Verification items for the finished model (mm, model axes). A direction names the side the tool comes from. Round coordinates to 2 decimals unless told otherwise and drop trailing zeros. Write each loop counter-clockwise with the first axis right and the second up, starting at its lowest first coordinate (ties: lowest second). Pieces come first, ordered by that corner, then holes. Notation, with made-up numbers: M 27,13.25 L 33,13.25 A24 ccw 33,42.25 Z; hole C 37.25,54.25 d1. An arc over 180 degrees is marked long. Answer in a Markdown table with one row per item. Add a question column.
1. Sectioned sample at B-B on z = 0. Record the cut outline in (x, y), plus the area to 3 significant figures.
2. Sectioned sample at A-A on y = 13.5. Record the cut outline in (x, z).
3. Sectioned sample at D-D on z = -7.5. Record the cut outline in (x, y), plus the area to 3 significant figures.
4. Sectioned sample at C-C on x = 0. Record the cut outline in (y, z), plus the area to 3 significant figures.
5. Go/stop test with flat-tipped pins: pin 1 Ø8 at (y, z) = (16.5, -6) entering from -X; pin 2 Ø1.6 at (y, z) = (15, 19.5) entering from +X; pin 3 Ø5 at (x, y) = (-17, 12) entering from +Z; pin 4 Ø12 at (x, z) = (6.5, -10) entering from -Y. Record where each tip stops, or that it passes through.
6. Material ranges on probe 1 along X at (y, z) = (31.05, 0); probe 2 along X at (y, z) = (8.5, 0); probe 3 along X at (y, z) = (25, 2.5), recorded low to high.
7. Set-up check for faces 1 (the flat face through (0, 0, 0)), 2 (the flat face through (-6, 16, 13.16)), 3 (the flat face through (-4.28, 30, 20)): record each of +Z, -Z, +X, -X, +Y, -Y from which the full face is reachable in a straight line by a thin tool's end or side.
8. Draft check along Z on faces 4 (the flat face through (0, 16, 21.46)), 5 (the flat face through (0, 27.573, 20)), 6 (the cylindrical face through (0.642, 16.993, -14.586)). Enter one of: pulls with the +Z half, pulls with the -Z half, needs draft (parallel to the pull), parting line crosses it, or undercut.
```python
from build123d import *

# Parameters (mm, degrees)
SKETCH1_R           = 17
BOSS_EXTRUDE1_DEPTH = 32
SHELL1_T            = -2.4
SKETCH2_R           = 3.45
BOSS_EXTRUDE3_DEPTH = 3
SKETCH4_R           = 2.25
CUT_EXTRUDE1_DEPTH  = 3
SKETCH5_W           = 12.1
SKETCH5_H           = 8.3
BOSS_EXTRUDE4_DEPTH = 26
SKETCH6_W           = 10.4
SKETCH6_H           = 8.6
CUT_EXTRUDE2_DEPTH  = 25
SKETCH7_W           = 8.6
SKETCH7_H           = 5.8
CUT_EXTRUDE3_DEPTH  = 5


with BuildPart() as part:
    # Sketch1 → Boss-Extrude1 (new body)
    with BuildSketch(Plane(origin=(0, 0, 0), x_dir=(1, 0, 0), z_dir=(0, 1, 0))):
        with Locations(Location((0, 0, 0), (0, 0, 270))):
            Circle(SKETCH1_R)
    extrude(amount=BOSS_EXTRUDE1_DEPTH)

    # Shell1
    shell1_openings = [part.faces().sort_by_distance(p)[0] for p in [
        (0, 32, 0),
    ]]
    offset(amount=SHELL1_T, openings=shell1_openings, kind=Kind.INTERSECTION)

    # Sketch2 → Boss-Extrude3 (add)
    with BuildSketch(Plane(origin=(0, 32, 0), x_dir=(1, 0, 0), z_dir=(0, 1, 0))):
        with Locations((18.659372003, 0)):
            Circle(SKETCH2_R)
        with Locations((-18.659372003, 0)):
            Circle(SKETCH2_R)
    extrude(amount=-BOSS_EXTRUDE3_DEPTH)

    # Sketch4 → Cut-Extrude1 (cut)
    with BuildSketch(Plane(origin=(0, 32, 0), x_dir=(1, 0, 0), z_dir=(0, 1, 0))):
        with Locations(Location((18.946509427, 0, 0), (0, 0, 270))):
            Circle(SKETCH4_R)
        with Locations(Location((-18.946509427, 0, 0), (0, 0, 331.648790534))):
            Circle(SKETCH4_R)
    extrude(amount=-CUT_EXTRUDE1_DEPTH, mode=Mode.SUBTRACT)

    # Sketch5 → Boss-Extrude4 (add)
    with BuildSketch(Plane(origin=(0, 32, 0), x_dir=(1, 0, 0), z_dir=(0, 1, 0))):
        with Locations((-0.271875844, -17.310314807)):
            Rectangle(SKETCH5_W, SKETCH5_H)
    extrude(amount=-BOSS_EXTRUDE4_DEPTH)

    # Sketch6 → Cut-Extrude2 (cut)
    with BuildSketch(Plane(origin=(0, 32, 0), x_dir=(1, 0, 0), z_dir=(0, 1, 0))):
        with Locations((0.116623003, -15.189562959)):
            Rectangle(SKETCH6_W, SKETCH6_H)
    extrude(amount=-CUT_EXTRUDE2_DEPTH, mode=Mode.SUBTRACT)

    # Sketch7 → Cut-Extrude3 (cut)
    with BuildSketch(Plane.XY.offset(21.460314807)):
        with Locations((0.019518241, 30.472573952)):
            Rectangle(SKETCH7_W, SKETCH7_H)
    extrude(amount=-CUT_EXTRUDE3_DEPTH, mode=Mode.SUBTRACT)


solid = part.part
```
Geometry check:
| question | item | result |
|---|---|---|
| 1 | outline | M -22.11,29 L -21.2,29 L -21.2,32 L -22.11,32 Z; M -17,0 L 17,0 L 17,29 L 16.7,29 L 16.7,32 L 14.6,32 L 14.6,2.4 L -14.6,2.4 L -14.6,32 L -16.7,32 L -16.7,29 L -17,29 Z; M 21.2,29 L 22.11,29 L 22.11,32 L 21.2,32 Z |
| 1 | area | 227 mm2 |
| 2 | outline | M -6.32,15.78 A17 ccw long 5.78,15.99 L 5.78,21.46 L -6.32,21.46 Z; hole M -6.32,13.16 A14.6 ccw long 5.78,13.41 L 5.78,13.16 L 5.32,13.16 L 5.32,19.49 L -5.08,19.49 L -5.08,13.16 Z |
| 3 | outline | M -15.26,0 L 15.26,0 L 15.26,32 L 12.53,32 L 12.53,2.4 L -12.53,2.4 L -12.53,32 L -15.26,32 Z |
| 3 | area | 235 mm2 |
| 4 | outline | M 0,-17 L 32,-17 L 32,-14.6 L 2.4,-14.6 L 2.4,14.6 L 6,14.6 L 6,13.16 L 7,13.16 L 7,19.49 L 27.57,19.49 L 27.57,21.46 L 6,21.46 L 6,17 L 0,17 Z |
| 4 | area | 210 mm2 |
| 5 | pin 1 | stops at x = -16.88 |
| 5 | pin 2 | stops at x = 5.78 |
| 5 | pin 3 | stops at z = 8.87 |
| 5 | pin 4 | stops at y = 0 |
| 6 | probe 1 | x = -22.11 to -21.2, -16.7 to -14.6, 14.6 to 16.7, 21.2 to 22.11 |
| 6 | probe 2 | x = -17 to -14.6, 14.6 to 17 |
| 6 | probe 3 | x = -16.82 to -14.38, 14.38 to 16.82 |
| 7 | face 1 | +Z, -Z, +X, -X, -Y |
| 7 | face 2 | +Y |
| 7 | face 3 | +Z, +Y |
| 8 | face 4 | pulls with the +Z half |
| 8 | face 5 | needs draft |
| 8 | face 6 | undercut |
